The model under review builds one solid part; all positions refer to its coordinate system, in mm. A direction names the side the tool comes from. Round coordinates to 2 decimals unless told otherwise and drop trailing zeros. Order: outer loops, then holes, each group sorted by start corner. A loop starts at its lowest first (then second) coordinate and runs counter-clockwise, first axis right, second up.
```python
from build123d import *

# Parameters (mm, degrees)
F0_W      = 40
F0_H      = 30
F1_DEPTH  = 5
F2_W      = 10
F2_H      = 10
F3_DEPTH  = 25
F4_W      = 5
F4_H      = 30
F5_DEPTH  = 28
F6_W      = 30
F6_H      = 5
F7_DEPTH  = 20
F8_R      = 4.99999
F9_R      = 2
F10_R     = 1.75
F11_DEPTH = 25


# Not quite as in the source:
# - a fillet or chamfer is up to 0.001 mm smaller than in the source, because OpenCascade refuses the exact size


with BuildPart() as f1:
    # F0 (on Top) → F1 (new body)
    with BuildSketch(Plane.XY):
        Rectangle(F0_W, F0_H)
    extrude(amount=F1_DEPTH)

    # F2 (on face) → F3 (cut)
    with BuildSketch(Plane.XY.offset(5)):
        with Locations((-15, 0)):
            Rectangle(F2_W, F2_H)
    extrude(amount=-F3_DEPTH, mode=Mode.SUBTRACT)

    # F4 (on face) → F5 (join)
    with BuildSketch(Plane(origin=(0, 0, 0), x_dir=(1, 0, 0), z_dir=(0, 0, -1))):
        with Locations((17.5, 0)):
            Rectangle(F4_W, F4_H)
    extrude(amount=F5_DEPTH)

    # F6 (on face) → F7 (join)
    with BuildSketch(Plane.YZ.offset(20)):
        with Locations((0, -25.5)):
            Rectangle(F6_W, F6_H)
    extrude(amount=F7_DEPTH)

    # F8 (radius 5 in the source; OpenCascade refuses exactly that, so slightly less here)
    f8_edges = [f1.edges().sort_by_distance(p)[0] for p in [
        (-20, 5, 2.5),
        (-20, -5, 2.5),
        (-20, -15, 2.5),
        (-20, 15, 2.5),
        (20, 0, 5),
        (-10, -5, 2.5),
        (-10, 5, 2.5),
        (15, 0, 0),
    ]]
    fillet(f8_edges, radius=F8_R)

    # F9
    f9_edges = [f1.edges().sort_by_distance(p)[0] for p in [
        (0, -15, 5),
        (-18.535537, -13.535537, 5),
        (15.00001, 0, 5),
        (-20, -10, 5),
        (0, 15, 5),
        (-18.535537, -6.464463, 5),
        (-18.535537, 13.535537, 5),
        (-15, -5, 5),
        (-20, 10, 5),
        (-11.464463, -3.535537, 5),
        (-18.535537, 6.464463, 5),
        (-10, 0, 5),
        (-15, 5, 5),
        (-11.464463, 3.535537, 5),
        (15, -15, -16.499995),
        (15, 0, -28),
        (-15.00001, -15, 2.5),
        (18.535537, -15, 3.535537),
        (-2.5, -15, 0),
        (20, -15, -11.499995),
        (13.535537, -15, -1.464463),
        (30, -15, -23),
        (40, -15, -25.5),
        (27.5, -15, -28),
        (20, 15, -11.499995),
        (18.535537, 15, 3.535537),
        (30, 15, -23),
        (40, 15, -25.5),
        (-15.00001, 15, 2.5),
        (27.5, 15, -28),
        (-2.5, 15, 0),
        (15, 15, -16.499995),
        (13.535537, 15, -1.464463),
    ]]
    fillet(f9_edges, radius=F9_R)

    # F10 (on face) → F11 (cut)
    with BuildSketch(Plane.XY.offset(-23)):
        with Locations((30, -8)):
            Circle(F10_R)
        with Locations((30, 8)):
            Circle(F10_R)
    extrude(amount=-F11_DEPTH, mode=Mode.SUBTRACT)


solid = f1.part
```
(1) Consider section A-A (x = 30). Write out the cut boundary in (y, z), and give its area (3 significant figures).
Data:
outline: (-15, -26) arc R2 ccw to (-13, -28) - (-9.75, -28) - (-9.75, -23) - (-13, -23) arc R2 ccw to (-15, -25) - close; (-6.25, -28) - (6.25, -28) - (6.25, -23) - (-6.25, -23) - close; (9.75, -28) - (13, -28) arc R2 ccw to (15, -26) - (15, -25) arc R2 ccw to (13, -23) - (9.75, -23) - close
area: 112 mm2
(2) Insertion check: pin 1 (4 mm diameter, centred on x = 30, y = -8, fed in from +Z); pin 2 (17 mm diameter, centred on y = 3.5, z = -17, fed in from -X); pin 3 (8 mm diameter, centred on x = 1.5, y = 2, fed in from -Z); pin 4 (12 mm diameter, centred on x = 5, z = -20, fed in from -Y). Each pin has a flat end and moves straight along its axis. Give the tip position at first contact, or say it passes through.
Data:
pin 1: stops at z = -23
pin 2: stops at x = 15
pin 3: stops at z = 0
pin 4: passes through
(3) For faces 4 (the cylindrical face through (-11.5, 3.57, 2.49)), 5 (the cylindrical face through (15.6, -14.43, -15.65)), 6 (the cylindrical face through (29.15, -14.43, -23.6)), list the 3-axis set-ups (+Z, -Z, +X, -X, +Y, -Y) from which the entire face can be reached by the end or side of a thin tool; tool diameter is ignored.
Data:
face 4: +Z, -Z, -X
face 5: -Z, -X, -Y
face 6: +Z, +X, -Y
(4) Consider section B-B (z = -22). Write out the cut boundary in (x, y).
Data:
outline: (15, -13) arc R2 ccw to (17, -15) - (18, -15) arc R2 ccw to (20, -13) - (20, 13) arc R2 ccw to (18, 15) - (17, 15) arc R2 ccw to (15, 13) - close
(5) To check wall thickness, follow probe 1 along Y at (x, z) = (30, -26.25); probe 2 along Y at (x, z) = (30, -24.3); probe 3 along Z at (x, y) = (-12, -7.5). State the ranges of each line that lie inside material, in increasing order.
Data:
probe 1: y = -14.98 to -9.75, -6.25 to 6.25, 9.75 to 14.98
probe 2: y = -14.87 to -9.75, -6.25 to 6.25, 9.75 to 14.87
probe 3: z = 0 to 5
(6) Draft analysis for pull direction Y (two halves, no side actions). For faces 1 (the flat face through (-1, 0, 0)), 2 (the cylindrical face through (-2.68, 14.43, 0.6)), 3 (the cylindrical face through (28.25, -7.92, -25.46)), state which applies: pulls with the +Y half, pulls with the -Y half, needs draft (parallel to the pull), parting line crosses it, or undercut.
Data:
face 1: needs draft
face 2: pulls with the +Y half
face 3: undercut
